```python
from build123d import *

# Parameters (mm, degrees)
MODEL_R             = 2.1
BOSS_EXTRUDE1_DEPTH = 400


with BuildPart() as part:
    # Model → Boss-Extrude1 (new body)
    with BuildSketch(Plane.XY):
        with BuildLine():
            Line((19, 10), (-19, 10))
            ThreePointArc((-19, 10), (-19.707106781, 9.707106781), (-20, 9))
            Line((-20, 9), (-20, 3.3))
            ThreePointArc((-20, 3.3), (-19.912132034, 3.087867966), (-19.7, 3))
            Line((-19.7, 3), (-18.3, 3))
            ThreePointArc((-18.3, 3), (-18.087867966, 3.087867966), (-18, 3.3))
            Line((-18, 3.3), (-18, 6))
            Line((-18, 6), (-17.060660172, 6))
            Line((-17.060660172, 6), (-14, 2.939339828))
            Line((-14, 2.939339828), (-14, 0.653589838))
            ThreePointArc((-14, 0.653589838), (-13.982962913, 0.524180316), (-13.933012702, 0.403589838))
            Line((-13.933012702, 0.403589838), (-13.7, 0))
            Line((-13.7, 0), (-13.933012702, -0.403589838))
            ThreePointArc((-13.933012702, -0.403589838), (-14, -0.653589838), (-13.933012702, -0.903589838))
            Line((-13.933012702, -0.903589838), (-13.750976592, -1.218885629))
            Line((-13.750976592, -1.218885629), (-14, -2.5))
            Line((-14, -2.5), (-14, -2.939339828))
            Line((-14, -2.939339828), (-17.060660172, -6))
            Line((-17.060660172, -6), (-18, -6))
            Line((-18, -6), (-18, -3.3))
            ThreePointArc((-18, -3.3), (-18.087867966, -3.087867966), (-18.3, -3))
            Line((-18.3, -3), (-19.7, -3))
            ThreePointArc((-19.7, -3), (-19.912132034, -3.087867966), (-20, -3.3))
            Line((-20, -3.3), (-20, -9))
            ThreePointArc((-20, -9), (-19.707106781, -9.707106781), (-19, -10))
            Line((-19, -10), (-13.3, -10))
            ThreePointArc((-13.3, -10), (-13.087867966, -9.912132034), (-13, -9.7))
            Line((-13, -9.7), (-13, -8.3))
            ThreePointArc((-13, -8.3), (-13.087867966, -8.087867966), (-13.3, -8))
            Line((-13.3, -8), (-16, -8))
            Line((-16, -8), (-16, -7.060660172))
            Line((-16, -7.060660172), (-12.939339828, -4))
            Line((-12.939339828, -4), (-10.653589838, -4))
            ThreePointArc((-10.653589838, -4), (-10.524180316, -3.982962913), (-10.403589838, -3.933012702))
            Line((-10.403589838, -3.933012702), (-10, -3.7))
            Line((-10, -3.7), (-9.596410162, -3.933012702))
            ThreePointArc((-9.596410162, -3.933012702), (-9.346410162, -4), (-9.096410162, -3.933012702))
            Line((-9.096410162, -3.933012702), (-8.781114371, -3.750976592))
            Line((-8.781114371, -3.750976592), (-7.5, -4))
            Line((-7.5, -4), (-7.060660172, -4))
            Line((-7.060660172, -4), (-4, -7.060660172))
            Line((-4, -7.060660172), (-4, -8))
            Line((-4, -8), (-6.7, -8))
            ThreePointArc((-6.7, -8), (-6.912132034, -8.087867966), (-7, -8.3))
            Line((-7, -8.3), (-7, -9.7))
            ThreePointArc((-7, -9.7), (-6.912132034, -9.912132034), (-6.7, -10))
            Line((-6.7, -10), (6.7, -10))
            ThreePointArc((6.7, -10), (6.912132034, -9.912132034), (7, -9.7))
            Line((7, -9.7), (7, -8.3))
            ThreePointArc((7, -8.3), (6.912132034, -8.087867966), (6.7, -8))
            Line((6.7, -8), (4, -8))
            Line((4, -8), (4, -7.060660172))
            Line((4, -7.060660172), (7.060660172, -4))
            Line((7.060660172, -4), (9.346410162, -4))
            ThreePointArc((9.346410162, -4), (9.475819684, -3.982962913), (9.596410162, -3.933012702))
            Line((9.596410162, -3.933012702), (10, -3.7))
            Line((10, -3.7), (10.403589838, -3.933012702))
            ThreePointArc((10.403589838, -3.933012702), (10.653589838, -4), (10.903589838, -3.933012702))
            Line((10.903589838, -3.933012702), (11.218885629, -3.750976592))
            Line((11.218885629, -3.750976592), (12.5, -4))
            Line((12.5, -4), (12.939339828, -4))
            Line((12.939339828, -4), (16, -7.060660172))
            Line((16, -7.060660172), (16, -8))
            Line((16, -8), (13.3, -8))
            ThreePointArc((13.3, -8), (13.087867966, -8.087867966), (13, -8.3))
            Line((13, -8.3), (13, -9.7))
            ThreePointArc((13, -9.7), (13.087867966, -9.912132034), (13.3, -10))
            Line((13.3, -10), (19, -10))
            ThreePointArc((19, -10), (19.707106781, -9.707106781), (20, -9))
            Line((20, -9), (20, -3.3))
            ThreePointArc((20, -3.3), (19.912132034, -3.087867966), (19.7, -3))
            Line((19.7, -3), (18.3, -3))
            ThreePointArc((18.3, -3), (18.087867966, -3.087867966), (18, -3.3))
            Line((18, -3.3), (18, -6))
            Line((18, -6), (17.060660172, -6))
            Line((17.060660172, -6), (14, -2.939339828))
            Line((14, -2.939339828), (14, -0.653589838))
            ThreePointArc((14, -0.653589838), (13.982962913, -0.524180316), (13.933012702, -0.403589838))
            Line((13.933012702, -0.403589838), (13.7, 0))
            Line((13.7, 0), (13.933012702, 0.403589838))
            ThreePointArc((13.933012702, 0.403589838), (14, 0.653589838), (13.933012702, 0.903589838))
            Line((13.933012702, 0.903589838), (13.750976592, 1.218885629))
            Line((13.750976592, 1.218885629), (14, 2.5))
            Line((14, 2.5), (14, 2.939339828))
            Line((14, 2.939339828), (17.060660172, 6))
            Line((17.060660172, 6), (18, 6))
            Line((18, 6), (18, 3.3))
            ThreePointArc((18, 3.3), (18.087867966, 3.087867966), (18.3, 3))
            Line((18.3, 3), (19.7, 3))
            ThreePointArc((19.7, 3), (19.912132034, 3.087867966), (20, 3.3))
            Line((20, 3.3), (20, 9))
            ThreePointArc((20, 9), (19.707106781, 9.707106781), (19, 10))
        make_face()
        with Locations((-10, 0)):
            Circle(MODEL_R, mode=Mode.SUBTRACT)
        with Locations((10, 0)):
            Circle(MODEL_R, mode=Mode.SUBTRACT)
        with BuildLine():
            Line((-8.5, 4), (-12.939339828, 4))
            Line((-12.939339828, 4), (-16, 7.060660172))
            Line((-16, 7.060660172), (-16, 8))
            Line((-16, 8), (-8.5, 8))
            ThreePointArc((-8.5, 8), (-7.792893219, 7.707106781), (-7.5, 7))
            Line((-7.5, 7), (-7.5, 5))
            ThreePointArc((-7.5, 5), (-7.792893219, 4.292893219), (-8.5, 4))
        make_face(mode=Mode.SUBTRACT)
        with BuildLine():
            Line((8.5, 4), (12.939339828, 4))
            Line((12.939339828, 4), (16, 7.060660172))
            Line((16, 7.060660172), (16, 8))
            Line((16, 8), (8.5, 8))
            ThreePointArc((8.5, 8), (7.792893219, 7.707106781), (7.5, 7))
            Line((7.5, 7), (7.5, 5))
            ThreePointArc((7.5, 5), (7.792893219, 4.292893219), (8.5, 4))
        make_face(mode=Mode.SUBTRACT)
        with BuildLine():
            Line((-6, 7), (-6, -2.939339828))
            Line((-6, -2.939339828), (-2.087867966, -6.851471863))
            ThreePointArc((-2.087867966, -6.851471863), (-2.02283614, -6.948798867), (-2, -7.063603897))
            Line((-2, -7.063603897), (-2, -7.7))
            ThreePointArc((-2, -7.7), (-1.912132034, -7.912132034), (-1.7, -8))
            Line((-1.7, -8), (1.7, -8))
            ThreePointArc((1.7, -8), (1.912132034, -7.912132034), (2, -7.7))
            Line((2, -7.7), (2, -7.063603897))
            ThreePointArc((2, -7.063603897), (2.02283614, -6.948798867), (2.087867966, -6.851471863))
            Line((2.087867966, -6.851471863), (6, -2.939339828))
            Line((6, -2.939339828), (6, 7))
            ThreePointArc((6, 7), (5.707106781, 7.707106781), (5, 8))
            Line((5, 8), (-5, 8))
            ThreePointArc((-5, 8), (-5.707106781, 7.707106781), (-6, 7))
        make_face(mode=Mode.SUBTRACT)
    extrude(amount=BOSS_EXTRUDE1_DEPTH)


solid = part.part
```
Design review of the part built by this model. Coordinates are the model's own, in mm. A direction names the side the tool comes from. Coordinates: 2 decimals unless noted, no trailing zeros.
1) Clearance check with flat-ended pins moving along their axes: pin 1 (3 mm diameter, centred on y = 1, z = 161, fed in from +X); pin 2 (12 mm diameter, centred on x = -8.5, y = 1.5, fed in from -Z); pin 3 (0.7 mm diameter, centred on x = -11.5, z = 172.5, fed in from -Y). State where each tip first meets the part, or that it passes through.
2) Mouldability with a two-part tool opening along Y and no side actions: class faces 3 (the flat face through (-12, 8, 197)), 4 (the flat face through (-9.2, 2.4, 400)), 5 (the flat face through (0, 8, 197)), 6 (the flat face through (0, -10, 197)) as +Y half, -Y half, draft (parallel to the pull), parting line (faces both ways), or undercut.
3) Wall thickness on line 1 along Y through (x, z) = (-10, 260.5); line 2 along Y through (x, z) = (-5, 188); line 3 along X through (y, z) = (5, 309): over which ranges is each line inside the solid? List them lowest first.
4) For faces 1 (the flat face through (-9.2, 2.4, 0)), 2 (the flat face through (12, 8, 197)), list the 3-axis set-ups (+Z, -Z, +X, -X, +Y, -Y) from which the entire face can be reached by the end or side of a thin tool; tool diameter is ignored.
5) Take a section at A-A, the plane z = 172.5. State how many separate pieces and enclosed holes the cut face has, and give its area (3 significant figures).
Returned:
1. pin 1: stops at x = 14
1. pin 2: stops at z = 0
1. pin 3: stops at y = -4
2. face 3: undercut
2. face 4: draft
2. face 5: undercut
2. face 6: -Y half
3. line 1: y = -3.7 to -2.1, 2.1 to 4, 8 to 10
3. line 2: y = -10 to -8, -6.06 to -3.94, 8 to 10
3. line 3: x = -20 to -18, -16.06 to -13.94, -7.5 to -6, 6 to 7.5, 13.94 to 16.06, 18 to 20
4. face 1: -Z, +X, -X, +Y, -Y
4. face 2: +Z, -Z
5. separate pieces: 1
5. enclosed holes: 5
5. area: 342 mm2
